Geometry: final body of the model. Coordinates: model frame, mm. A direction names the side the tool comes from. Give positions to 0.01 mm unless a question says otherwise; leave off trailing zeros. Write each loop counter-clockwise with the first axis right and the second up, starting at its lowest first coordinate (ties: lowest second). Pieces come first, ordered by that corner, then holes.
Q1. Cut plane A-A on x = 0. Return the cut outline in (y, z).
Q2. Cut plane D-D on x = -7.5. Return the cut outline in (y, z).
Q3. Line query: L1, parallel to X at y = 4.8, z = 2.25; L2, parallel to Y at x = 9.75, z = 3.5; L3, parallel to Z at x = 0, y = 3.15. Output: solid intervals per line, ascending.
Q4. Draft query along Z for faces 1 (the face through (10, 1.2, -3.2)), 2 (the face through (-9.5, 1.27, -0.07)), 3 (the face through (5, 0, 0)). Return one class per face: pulls with the +Z half, pulls with the -Z half, needs draft (parallel to the pull), parting line crosses it, or undercut.
Q5. Pin query (flat end, axial travel): pin 1 (4 mm diameter, centred on x = -8, z = 0, fed in from +Y). Return the tip coordinate at first contact, or that it passes through.
Q6. Cut plane B-B on z = 8.5. Return the cut outline in (x, y), plus the area to 3 significant figures.
Q7. Cut plane C-C on y = 0.7. Return the cut outline in (x, z), plus the area to 3 significant figures.
Q8. Reachability of faces 4 (the face through (0.07, 1.27, -9.5)), 5 (the face through (5, 2.5, 5)) from +Z, -Z, +X, -X, +Y, -Y: full face, straight path, thin tool, end or side. Return the list, or none.
```python
from build123d import *

# Parameters (mm, degrees)
SKETCH_1_R               = 10.5
SKETCH_1_R_2             = 4.4
EXTRUDE_1_DEPTH          = 2.5
SKETCH_2_R               = 5.5
SKETCH_2_R_2             = 4.4
EXTRUDE_2_DEPTH          = 2.5
SKETCH_3_R               = 1.5
CUT_EXTRUDE_1_DEPTH      = 3.5
PATTERN_CIRCULAR_2_COUNT = 4


with BuildPart() as part:
    # Эскиз1 → Бобышка-Вытянуть1 (new body)
    with BuildSketch(Plane(origin=(0, 0, 0), x_dir=(1, 0, 0), z_dir=(0, 1, 0))):
        Circle(SKETCH_1_R)
        Circle(SKETCH_1_R_2, mode=Mode.SUBTRACT)
    extrude(amount=EXTRUDE_1_DEPTH)

    # Эскиз2 → Бобышка-Вытянуть2 (add)
    with BuildSketch(Plane(origin=(0, 2.5, 0), x_dir=(1, 0, 0), z_dir=(0, 1, 0))):
        Circle(SKETCH_2_R)
        Circle(SKETCH_2_R_2, mode=Mode.SUBTRACT)
    extrude(amount=EXTRUDE_2_DEPTH)

    # Эскиз3 → Вырез-Вытянуть1 (cut, through all)
    with BuildSketch(Plane(origin=(0, 2.5, 0), x_dir=(1, 0, 0), z_dir=(0, 1, 0))):
        with Locations((-8, 0)):
            Circle(SKETCH_3_R)
    cut_extrude_1 = extrude(amount=-CUT_EXTRUDE_1_DEPTH, mode=Mode.SUBTRACT)

    # Круговой массив2: Вырез-Вытянуть1 ×4 about axis
    pattern_circular_2_axis = Axis((0, 0, 0), (0, 1, 0))
    for i in range(1, PATTERN_CIRCULAR_2_COUNT):
        add(cut_extrude_1.rotate(pattern_circular_2_axis, i * 360 / PATTERN_CIRCULAR_2_COUNT), mode=Mode.SUBTRACT)


solid = part.part
```
Data:
1. outline: (0, -10.5) - (2.5, -10.5) - (2.5, -9.5) - (0, -9.5) - close; (0, -6.5) - (2.5, -6.5) - (2.5, -5.5) - (5, -5.5) - (5, -4.4) - (0, -4.4) - close; (0, 4.4) - (5, 4.4) - (5, 5.5) - (2.5, 5.5) - (2.5, 6.5) - (0, 6.5) - close; (0, 9.5) - (2.5, 9.5) - (2.5, 10.5) - (0, 10.5) - close
2. outline: (0, -7.35) - (2.5, -7.35) - (2.5, -1.41) - (0, -1.41) - close; (0, 1.41) - (2.5, 1.41) - (2.5, 7.35) - (0, 7.35) - close
3. L1: x = -5.02 to -3.78, 3.78 to 5.02
3. L2: y = 0 to 2.5
3. L3: z = -5.5 to -4.4, 4.4 to 5.5
4. face 1: parting line crosses it
4. face 2: undercut
4. face 3: needs draft
5. pin 1: stops at y = 2.5
6. outline: (-6.16, 0) - (-1.41, 0) - (-1.41, 2.5) - (-6.16, 2.5) - close; (1.41, 0) - (6.16, 0) - (6.16, 2.5) - (1.41, 2.5) - close
6. area: 23.8 mm2
7. outline: circle Ø21 at (0, 0); hole circle Ø3 at (-8, 0); hole circle Ø8.8 at (0, 0); hole circle Ø3 at (0, -8); hole circle Ø3 at (0, 8); hole circle Ø3 at (8, 0)
7. area: 257 mm2
8. face 4: +Y, -Y
8. face 5: +Y
